Input: dimensioned drawing with shaded views. Units: mm. Origin: part minimum x, y, z. Round coordinates to 2 decimals unless told otherwise and drop trailing zeros. Order: outer loops, then holes, each group sorted by start corner. A loop starts at its lowest first (then second) coordinate and runs counter-clockwise, first axis right, second up. Notation, with made-up numbers: (-8, -13) - (29, -13) arc R38 cw to (29, 26) - close; hole circle Ø1 at (65.5, 38.25). An arc over 180 degrees is marked (long way). Return JSON: item names as keys, results as strings. Group by question number.
1) Section A-A, the plane x = 65. Return loops of the section in (y, z).
2) Section C-C, the plane y = 107.5. Return loops of the section in (x, z), plus the area to 3 significant figures.
3) Contact query for flat-ended pins moving along their axis: P1, Ø10, axis at x = 26.11, y = 103.89, coming from the +Z side; P2, Ø1, axis at x = 98, z = 2.5, coming from the +Y side. Output: stop coordinate, or through.
4) Ray query, line 1 (Y direction, x = 63.5, z = 2.45); line 2 (X direction, y = 55, z = 0.5); line 3 (X direction, y = 26, z = 0.3). Return the intervals inside material, ascending. Write a range as from..to.
5) Section D-D, the plane z = 1.6. Return loops of the section in (x, y), plus the area to 3 significant figures.
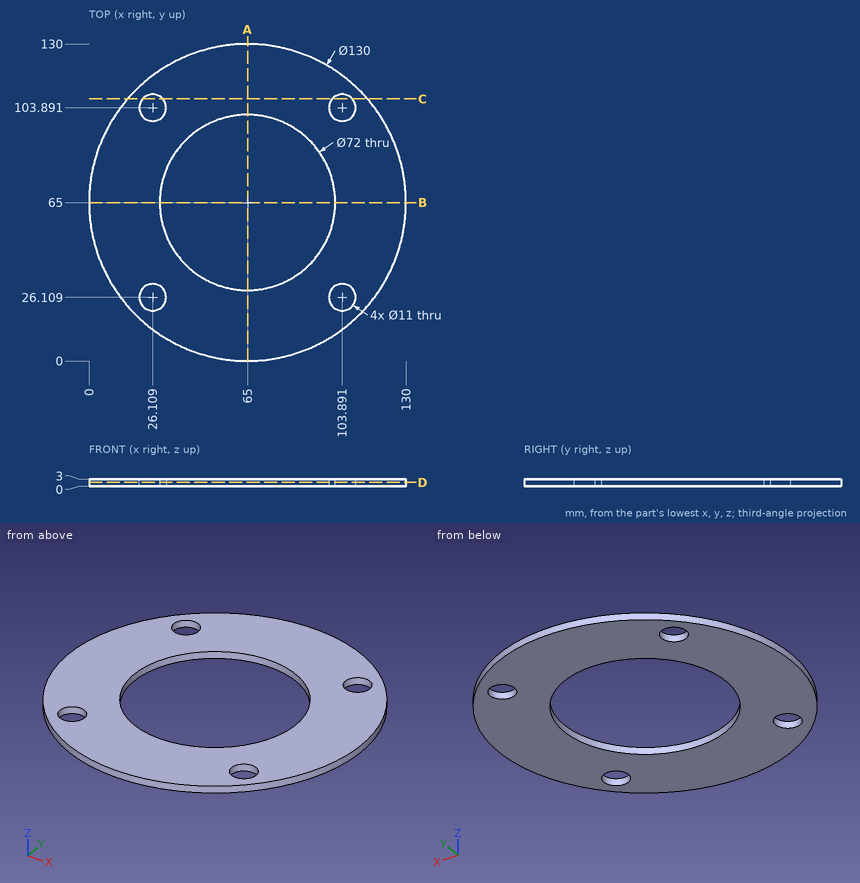
Geometry check:
{
 "1": {"outline": "(0, 0) - (29, 0) - (29, 3) - (0, 3) - close; (101, 0) - (130, 0) - (130, 3) - (101, 3) - close"},
 "2": {"outline": "(15.82, 0) - (21.96, 0) - (21.96, 3) - (15.82, 3) - close; (30.26, 0) - (99.74, 0) - (99.74, 3) - (30.26, 3) - close; (108.04, 0) - (114.18, 0) - (114.18, 3) - (108.04, 3) - close", "area": "245 mm2"},
 "3": {"P1": "through", "P2": "y = 121.29"},
 "4": {"line 1": "0.02..29.03, 100.97..129.98", "line 2": "0.77..30.42, 99.58..129.23", "line 3": "13..20.61, 31.61..98.39, 109.39..117"},
 "5": {"outline": "circle Ø130 at (65, 65); hole circle Ø11 at (26.11, 26.11); hole circle Ø11 at (26.11, 103.89); hole circle Ø72 at (65, 65); hole circle Ø11 at (103.89, 26.11); hole circle Ø11 at (103.89, 103.89)", "area": "8,820 mm2"}
}
